Verification items for the finished model (mm, model axes). A direction names the side the tool comes from. Coordinates: 2 decimals unless noted, no trailing zeros. Loops run counter-clockwise (first coordinate to the right, second up) from the corner with the lowest first, then second, coordinate; pieces in that order, holes last. Notation, with made-up numbers: (68, -32.75) - (90, -32.75) arc R20 ccw to (90, -18.75) - close; hole circle Ø2 at (22.5, -25.75). An arc over 180 degrees is marked (long way). Answer as CSV lines item,"result". Start each with the question number.
1. Cross-section at D-D (x = -10.25). Enter the section's corners in (y, z).
2. Material ranges on line 1 (Z direction, x = -11.5, y = 14.25); line 2 (Y direction, x = 8.5, z = -4); line 3 (Y direction, x = -7.5, z = -2.3), recorded low to high. Write a range as [from, to].
3. Cross-section at A-A (y = 6.5). Enter the section's corners in (x, z), plus the area to 3 significant figures.
4. Gauge pin test, flat ends, axial feed: P1, Ø4, axis at x = 7.5, y = 9, coming from the +Z side; P2, Ø5, axis at x = 4, z = -8.5, coming from the +Y side; P3, Ø1.5, axis at x = -3.5, z = 8.5, coming from the -Y side; P4, Ø4, axis at x = -7.5, y = 9, coming from the -Z side. Record the tip position at first contact, or that the pin passes through.
5. Set-up check for faces 5 (the flat face through (0, 1, -12.5)), 6 (the flat face through (-9, 8, -1)), 7 (the flat face through (-3.5, 9, -2)), 8 (the flat face through (-9, 8, -3)): record each of +Z, -Z, +X, -X, +Y, -Y from which the full face is reachable in a straight line by a thin tool's end or side.
6. Cross-section at C-C (y = 9). Enter the section's corners in (x, z).
7. Cross-section at B-B (z = 0). Enter the section's corners in (x, y), plus the area to 3 significant figures.
8. Release check for a two-part mould opening along X. For faces 1 (the cylindrical face through (6.084, 1.479, 7.409)), 2 (the flat face through (-12.5, 2, -1)), 3 (the flat face through (-8, 15, -2)), 4 (the flat face through (3.5, 9, -2)) record: pulls with the +X half, pulls with the -X half, needs draft (parallel to the pull), parting line crosses it, or undercut.
```python
from build123d import *

# Parameters (mm, degrees)
SKETCH4_W           = 25
SKETCH4_H           = 25
BOSS_EXTRUDE2_DEPTH = 3
SKETCH1_R           = 1.75
CUT_EXTRUDE3_DEPTH  = 18.930421077
SKETCH5_W           = 9
SKETCH5_H           = 2
BOSS_EXTRUDE3_DEPTH = 12
SKETCH6_R           = 3.25
CUT_EXTRUDE4_DEPTH  = 24.184046239
SKETCH7_R           = 1.5
CUT_EXTRUDE5_DEPTH  = 2


with BuildPart() as part:
    # Sketch4 → Boss-Extrude2 (new body)
    with BuildSketch(Plane(origin=(0, 0, 0), x_dir=(1, 0, 0), z_dir=(0, 1, 0))):
        Rectangle(SKETCH4_W, SKETCH4_H)
    extrude(amount=BOSS_EXTRUDE2_DEPTH)

    # Sketch1 → Cut-Extrude3 (cut, through all)
    with BuildSketch(Plane(origin=(0, 0, 0), x_dir=(1, 0, 0), z_dir=(0, 1, 0))):
        with Locations(Location((-7.266656382, 6.119289585, 0), (0, 0, 270))):
            Circle(SKETCH1_R)
        with Locations(Location((5.153085966, 6.119289585, 0), (0, 0, 270))):
            Circle(SKETCH1_R)
        with Locations(Location((-5.153085966, -6.119289585, 0), (0, 0, 90))):
            Circle(SKETCH1_R)
        with Locations(Location((7.266656382, -6.119289585, 0), (0, 0, 90))):
            Circle(SKETCH1_R)
    extrude(amount=CUT_EXTRUDE3_DEPTH, mode=Mode.SUBTRACT)

    # Sketch5 → Boss-Extrude3 (add)
    with BuildSketch(Plane(origin=(0, 3, 0), x_dir=(1, 0, 0), z_dir=(0, 1, 0))):
        with Locations((8, 2)):
            Rectangle(SKETCH5_W, SKETCH5_H)
        with Locations((-8, 2)):
            Rectangle(SKETCH5_W, SKETCH5_H)
    extrude(amount=BOSS_EXTRUDE3_DEPTH)

    # Sketch6 → Cut-Extrude4 (cut, through all)
    with BuildSketch(Plane.XZ):
        with Locations(Location((0, 0, 0), (0, 0, 270))):
            Circle(SKETCH6_R)
    extrude(amount=-CUT_EXTRUDE4_DEPTH, mode=Mode.SUBTRACT)

    # Sketch7 → Cut-Extrude5 (cut)
    with BuildSketch(Plane(origin=(0, 0, -3), x_dir=(-1, 0, 0), z_dir=(0, 0, -1))):
        with Locations((-7.5, 9)):
            Circle(SKETCH7_R)
        with Locations((7.5, 9)):
            Circle(SKETCH7_R)
    extrude(amount=-CUT_EXTRUDE5_DEPTH, mode=Mode.SUBTRACT)


solid = part.part
```
Values follow:
1,outline,"(0, -12.5) - (3, -12.5) - (3, -3) - (15, -3) - (15, -1) - (3, -1) - (3, 12.5) - (0, 12.5) - close"
2,line 1,"z = [-3, -1]"
2,line 2,"y = [0, 3]"
2,line 3,"y = [0, 7.5], [10.5, 15]"
3,outline,"(-12.5, -3) - (-3.5, -3) - (-3.5, -1) - (-12.5, -1) - close; (3.5, -3) - (12.5, -3) - (12.5, -1) - (3.5, -1) - close"
3,area,"36.0 mm²"
4,P1,"stops at z = -1"
4,P2,"stops at y = 3"
4,P3,"stops at y = 0"
4,P4,"stops at z = -3"
5,face 5,"-Z, +X, -X, +Y, -Y"
5,face 6,"+Z, +X, -X, +Y"
5,face 7,"+Z, -Z, +Y"
5,face 8,"-Z, +X, -X, +Y"
6,outline,"(-12.5, -3) - (-9, -3) - (-9, -1) - (-12.5, -1) - close; (-6, -3) - (-3.5, -3) - (-3.5, -1) - (-6, -1) - close; (3.5, -3) - (6, -3) - (6, -1) - (3.5, -1) - close; (9, -3) - (12.5, -3) - (12.5, -1) - (9, -1) - close"
7,outline,"(-12.5, 0) - (-3.25, 0) - (-3.25, 3) - (-12.5, 3) - close; (3.25, 0) - (12.5, 0) - (12.5, 3) - (3.25, 3) - close"
7,area,"55.5 mm²"
8,face 1,"undercut"
8,face 2,"pulls with the -X half"
8,face 3,"needs draft"
8,face 4,"undercut"
